from build123d import *

# Parameters (mm, degrees)
BOARD_DEPTH        = 1.68
SKETCH2_R          = 1.5
SKETCH2_R_2        = 0.4953
PLATED_HOLES_DEPTH = 5.7


with BuildPart() as part:
    # Sketch1 → BOARD (new body)
    with BuildSketch(Plane.XY.offset(-4.7)):
        with BuildLine():
            Line((100, 43), (100, 60.5))
            ThreePointArc((100, 60.5), (98.681980515, 63.681980515), (95.5, 65))
            Line((95.5, 65), (83, 65))
            ThreePointArc((83, 65), (80.878679656, 64.121320344), (80, 62))
            Line((80, 62), (80, 43))
            ThreePointArc((80, 43), (80.878679656, 40.878679656), (83, 40))
            Line((83, 40), (97, 40))
            ThreePointArc((97, 40), (99.121320344, 40.878679656), (100, 43))
        make_face()
    extrude(amount=BOARD_DEPTH)

    # Sketch2 → PLATED HOLES (cut, through all)
    with BuildSketch(Plane.XY):
        with Locations((83, 42.5)):
            Circle(SKETCH2_R)
        with Locations((97, 42.5)):
            Circle(SKETCH2_R)
        with Locations((97, 35.5)):
            Circle(SKETCH2_R)
        with Locations((83, 62)):
            Circle(SKETCH2_R)
        with Locations((87.749999989, 55.999999989)):
            Circle(SKETCH2_R_2)
        with Locations((87.749999989, 60.999999996)):
            Circle(SKETCH2_R_2)
        with Locations((94.000000011, 58.499999992)):
            Circle(SKETCH2_R_2)
        with Locations((94.000000011, 55.999999989)):
            Circle(SKETCH2_R_2)
        with Locations((94.000000011, 60.999999996)):
            Circle(SKETCH2_R_2)
    extrude(amount=-PLATED_HOLES_DEPTH, mode=Mode.SUBTRACT)


solid = part.part
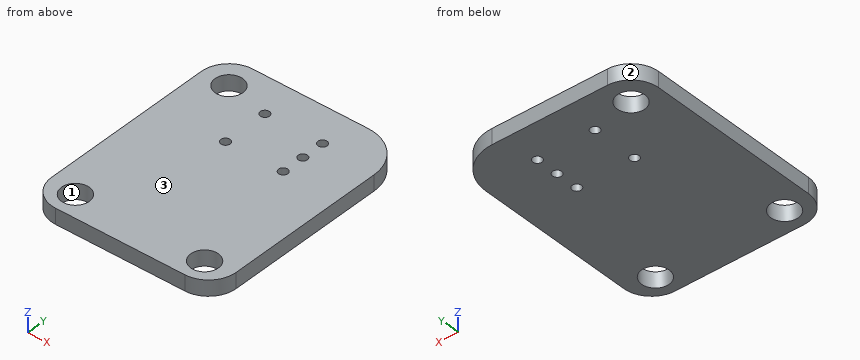
Part model, mm, in its own coordinate system. Face numbers are marked on the shaded views. Give positions to 0.01 mm unless a question says otherwise; leave off trailing zeros. Write each loop counter-clockwise with the first axis right and the second up, starting at its lowest first coordinate (ties: lowest second). Pieces come first, ordered by that corner, then holes.
1) Two-plate mould, pull along X, no slides. Class the marked faces 1, 2 and 3: released by +X, released by -X, zero draft, split by the parting line, or undercut.
Resolved:
face 1: undercut
face 2: released by -X
face 3: zero draft
2) Cut at C-C on y = 58.5. Write the cut outline in (x, z), then the cut area to 3 significant figures.
Resolved:
outline: (80, -4.7) - (93.5, -4.7) - (93.5, -3.02) - (80, -3.02) - close; (94.5, -4.7) - (100, -4.7) - (100, -3.02) - (94.5, -3.02) - close
area: 31.9 mm2
3) Cut at D-D on z = -3.7. State how many separate pieces and enclosed holes the cut face has, then the cut area to 3 significant figures.
Resolved:
separate pieces: 1
enclosed holes: 8
area: 465 mm2
4) Probe L1, parallel to Y at x = 83, z = -3.8; L2, parallel to Y at x = 94, z = -4.15; L3, parallel to Y at x = 87.75, z = -3.8. List the from-to ranges inside material, lowest first.
Resolved:
L1: y = 40 to 41, 44 to 60.5, 63.5 to 65
L2: y = 40 to 55.5, 56.5 to 58, 59 to 60.5, 61.5 to 65
L3: y = 40 to 55.5, 56.5 to 60.5, 61.5 to 65
5) Cut at A-A on x = 87.75. Write the cut outline in (y, z), then the cut area to 3 significant figures.
Resolved:
outline: (40, -4.7) - (55.5, -4.7) - (55.5, -3.02) - (40, -3.02) - close; (56.5, -4.7) - (60.5, -4.7) - (60.5, -3.02) - (56.5, -3.02) - close; (61.5, -4.7) - (65, -4.7) - (65, -3.02) - (61.5, -3.02) - close
area: 38.7 mm2
6) Cut at B-B on y = 56. Write the cut outline in (x, z).
Resolved:
outline: (80, -4.7) - (87.25, -4.7) - (87.25, -3.02) - (80, -3.02) - close; (88.25, -4.7) - (93.5, -4.7) - (93.5, -3.02) - (88.25, -3.02) - close; (94.5, -4.7) - (100, -4.7) - (100, -3.02) - (94.5, -3.02) - close
7) Pin check, flat tip, straight feed: pin 1 (5 mm diameter, centred on x = 97, y = 42.5, fed in from -Z). Stop position of the tip, or through.
Resolved:
pin 1: stops at z = -4.7
